Read the model definition and answer for the solid it produces. Units are mm, in the model's axes. A direction names the side the tool comes from. Give positions to 0.01 mm unless a question says otherwise; leave off trailing zeros. Order: outer loops, then holes, each group sorted by start corner. A loop starts at its lowest first (then second) coordinate and runs counter-clockwise, first axis right, second up. Notation, with made-up numbers: (52.25, 37) -> (80.25, 37) arc R6 cw to (80.25, 45) -> close; hole circle Ø7 at (0.5, -9.75). An arc over 180 degrees is marked (long way). One line per item, written item: value. Start each with the question number.
from build123d import *

# Parameters (mm, degrees)
F0_W     = 216.339796
F0_H     = 94.022334
F3_DEPTH = 25.4
F1_W     = 231.186748
F1_H     = 102.275074
F1_W_2   = 216.339796
F1_H_2   = 94.022334
F4_DEPTH = 50.8
F2_W     = 240.056262
F2_H     = 108.75938
F2_W_2   = 216.339796
F2_H_2   = 94.022334
F5_DEPTH = 127


with BuildPart() as f3:
    # F0 (on Top) → F3 (new body)
    with BuildSketch(Plane.XY):
        Rectangle(F0_W, F0_H)
    extrude(amount=F3_DEPTH)

    # F1 (on face) → F4 (join)
    with BuildSketch(Plane.XY):
        Rectangle(F1_W, F1_H)
        Rectangle(F1_W_2, F1_H_2, mode=Mode.SUBTRACT)
    extrude(amount=F4_DEPTH)

    # F2 (on face) → F5 (join)
    with BuildSketch(Plane.XY):
        Rectangle(F2_W, F2_H)
        Rectangle(F2_W_2, F2_H_2, mode=Mode.SUBTRACT)
    extrude(amount=F5_DEPTH)


solid = f3.part
Item 1: Find section A-A on x = 8. Write down the section's boundary in (y, z).
Item 2: A flat-ended cylindrical pin translates along its axis: pin 1 (4 mm diameter, centred on x = -45.5, y = 28.5, fed in from +Z). Find the tip coordinate at first contact, or state that the pin passes through.
Item 3: Find the intervals of material crossed by line 1 (Y direction, x = 81.5, z = 34.5); line 2 (X direction, y = -22.5, z = 65.5); line 3 (Z direction, x = 63, y = 16.5), in increasing order. Write a range as from..to.
Item 4: Find section C-C on y = -3.5. Write down the section's boundary in (x, z), then the cut area to 3 significant figures.
Item 5: For a pull along X with two mould halves and no side action, classify faces 3 (the flat face through (-9, -48, 127)), 4 (the flat face through (-120.028, -1, 63)), 5 (the flat face through (120.028, -1, 63)), 6 (the flat face through (-2, 47.011, 75)) as +X half, -X half, draft (parallel to the pull), parting line (faces both ways), or undercut.
Item 6: A tool of negligible diameter and unlimited length cuts with its end or side. For faces 1 (the flat face through (108.17, -1, 75)), 2 (the flat face through (-2, 1, 0)), from which of +Z, -Z, +X, -X, +Y, -Y can it reach the whole face along a straight path? Write none if from no direction.
Item 7: Find section B-B on z = 96.5. Write down the section's boundary in (x, y), then the cut area to 3 significant figures.
Checks:
1. outline: (-54.38, 0) -> (54.38, 0) -> (54.38, 127) -> (47.01, 127) -> (47.01, 25.4) -> (-47.01, 25.4) -> (-47.01, 127) -> (-54.38, 127) -> close
2. pin 1: z = 25.4
3. line 1: -54.38..-47.01, 47.01..54.38
3. line 2: -120.03..-108.17, 108.17..120.03
3. line 3: 0..25.4
4. outline: (-120.03, 0) -> (120.03, 0) -> (120.03, 127) -> (108.17, 127) -> (108.17, 25.4) -> (-108.17, 25.4) -> (-108.17, 127) -> (-120.03, 127) -> close
4. area: 8,510 mm2
5. face 3: draft
5. face 4: -X half
5. face 5: +X half
5. face 6: undercut
6. face 1: +Z
6. face 2: -Z, +X, -X, +Y, -Y
7. outline: (-120.03, -54.38) -> (120.03, -54.38) -> (120.03, 54.38) -> (-120.03, 54.38) -> close; hole (-108.17, -47.01) -> (108.17, -47.01) -> (108.17, 47.01) -> (-108.17, 47.01) -> close
7. area: 5,770 mm2
